Autodesk Inventor part; units mm, degrees
ref_plane "XZ Plane" through (0, 0, 0) normal (0, 1, 0) x (-1, 0, 0)
ref_plane "XY Plane" through (0, 0, 0) normal (0, 0, 1) x (1, 0, 0)
sketch "Sketch1" plane through (0, 0, 0) normal (0, 1, 0) x (-1, 0, 0)
  line L0 (0, 0) -> (0, -319.927) construction
  line L1 (-4, 0) -> (-4, -319.927)
  line L2 (4, -319.927) -> (4, 0)
  arc A0 (4, 0) -> (-4, 0) centre (0, 0) ccw
  arc A1 (-4, -319.927) -> (4, -319.927) centre (0, -319.927) ccw
  circle A2 centre (0, 0) radius 1.5
  circle A3 centre (0, -319.927) radius 1.5
  line L3 (0, -50.8) -> (0, -100) construction
  line L4 (-1.5, -50.8) -> (-1.5, -100)
  line L5 (1.5, -100) -> (1.5, -50.8)
  arc A4 (1.5, -50.8) -> (-1.5, -50.8) centre (0, -50.8) ccw
  arc A5 (-1.5, -100) -> (1.5, -100) centre (0, -100) ccw
  arc A6 (4, 0) -> (4, -40) centre (202.9975, -20) ccw
  arc A7 (-4, 0) -> (-4, -40) centre (194.9975, -20) ccw
  point P0 (0, -159.9635)
  point P1 (0, -75.4)
  dimension "d0" = 319.927
  dimension "d1" = 8
  dimension "d2" = 3
  dimension "d3" = 3
  dimension "d12" = 3
  dimension "d13" = 50.8
  dimension "d14" = 100
  dimension "d15" = 40
  dimension "d16" = 200
  dimension "d17" = 200
extrude "Extrusion1" add sketch "Sketch1" along normal blind 8 contours A0 A6 L2 A1 L1 | L1 A7
sketch "Sketch2" plane through (0, 0, 0) normal (0, -1, 0) x (1, 0, 0)
  arc A0 (4, -40) -> (4, 0) centre (-194.9975, -20) ccw
  arc A1 (4, 0) -> (-4, 0) centre (0, 0) ccw
  arc A2 (-4, -40) -> (-4, 0) centre (-202.9975, -20) ccw
  line L0 (-4, -319.927) -> (-4, -40)
  arc A3 (-4, -319.927) -> (4, -319.927) centre (0, -319.927) ccw
  line L1 (4, -40) -> (4, -319.927)
  circle A4 centre (0, 0) radius 1.5
  circle A5 centre (0, -319.927) radius 1.5
  arc A6 (1.5, -50.8) -> (-1.5, -50.8) centre (0, -50.8) ccw
  line L2 (1.5, -100) -> (1.5, -50.8)
  arc A7 (-1.5, -100) -> (1.5, -100) centre (0, -100) ccw
  line L3 (-1.5, -50.8) -> (-1.5, -100)
The listing builds one solid part. Answer for the finished solid, in the listing's coordinates (mm). A direction names the side the tool comes from. Give positions to 0.01 mm unless a question says otherwise; leave off trailing zeros. Loops run counter-clockwise (first coordinate to the right, second up) from the corner with the lowest first, then second, coordinate; pieces in that order, holes last. Notation, with made-up numbers: M 87.5,-32 L 119.5,-32 A15 cw 119.5,-4 Z; hole C 24,-12 d1. An arc over 180 degrees is marked long. One line per item, written item: value.
Q1. Determine the mould class of faces 1 (the face through (-1.5, 4, -76)), 2 (the face through (5.002, 3.944, -20.28)), 3 (the face through (-2.998, 3.944, -20.28)) for opening direction X: +X half, -X half, draft (parallel to the pull), parting line (faces both ways), or undercut.
Working result:
face 1: undercut
face 2: +X half
face 3: -X half
Q2. A cutting plane is placed at D-D on z = -260. Determine the outline of the cut face in (x, y).
Working result:
outline: M -4,0 L 4,0 L 4,8 L -4,8 Z
Q3. For faces 4 (the face through (0, 4, 4)), 5 (the face through (1.5, 4, -75)), 6 (the face through (4, 4, -178)), determine the directions among +Z, -Z, +X, -X, +Y, -Y from which every point of the face is accessible in a straight line to the end or side of a thin tool.
Working result:
face 4: +Z, +Y, -Y
face 5: +Y, -Y
face 6: -Z, +X, +Y, -Y
Q4. Flat-ended cylindrical pins translate along their axes: P1, Ø4, axis at x = 0, z = 0, coming from the +Y side; P2, Ø4, axis at y = 5, z = -135, coming from the +X side; P3, Ø2.5, axis at x = 0, z = -319.927, coming from the -Y side. Find the tip coordinate at first contact, or state that the pin passes through.
Working result:
P1: stops at y = 8
P2: stops at x = 4
P3: passes through
Q5. A cutting plane is placed at B-B on z = -84. Determine the outline of the cut face in (x, y).
Working result:
outline: M -4,0 L -1.5,0 L -1.5,8 L -4,8 Z; M 1.5,0 L 4,0 L 4,8 L 1.5,8 Z
Q6. Find the intervals of material crossed by line 1 (Z direction, x = 0, y = 4.5); line 2 (X direction, y = 7.25, z = -64); line 3 (X direction, y = 3.25, z = -242.5), in increasing order. Write a range as from..to.
Working result:
line 1: z = -323.93..-321.43, -318.43..-101.5, -49.3..-1.5, 1.5..4
line 2: x = -4..-1.5, 1.5..4
line 3: x = -4..4
Q7. A cutting plane is placed at A-A on y = 3. Determine the outline of the cut face in (x, z), then the cut area to 3 significant figures.
Working result:
outline: M -4,-319.93 A4 ccw 4,-319.93 L 4,-40 A200 ccw 4,0 A4 ccw -4,0 A200 cw -4,-40 Z; hole C 0,-319.93 d3; hole M -1.5,-100 A1.5 ccw 1.5,-100 L 1.5,-50.8 A1.5 ccw -1.5,-50.8 Z; hole C 0,0 d3
area: 2,440 mm^2
Q8. A cutting plane is placed at C-C on x = 0. Determine the outline of the cut face in (y, z).
Working result:
outline: M 0,-323.93 L 8,-323.93 L 8,-321.43 L 0,-321.43 Z; M 0,-318.43 L 8,-318.43 L 8,-101.5 L 0,-101.5 Z; M 0,-49.3 L 8,-49.3 L 8,-1.5 L 0,-1.5 Z; M 0,1.5 L 8,1.5 L 8,4 L 0,4 Z
